Geometry: final body of the model. Coordinates: model frame, mm. Face numbers are marked on the shaded views. A direction names the side the tool comes from. Coordinates: 2 decimals unless noted, no trailing zeros. Order: outer loops, then holes, each group sorted by start corner. A loop starts at its lowest first (then second) coordinate and runs counter-clockwise, first axis right, second up. Notation, with made-up numbers: M 19,29 L 51,29 A14 ccw 51,52 Z; hole C 84,30.5 d10. An arc over 180 degrees is marked long. Use CSV: the item, a comma, the result in double quotes. Start each with the question number.
Q1. Section query C-C, the plane y = 33.5. Output: boundary loops of the cut face in (x, z).
Q2. Mould query, pull axis X, two halves, no side actions, for the marked faces 1, 2 and 3. Classes: +X half, -X half, draft (parallel to the pull), parting line (faces both ways), or undercut.
Q3. Access query for the marked faces 4 and 5. Directions: +Z, -Z, +X, -X, +Y, -Y. A direction counts if a zero-diameter tool reaches every point of the face in a straight line with its end or side. Return the directions, or none.
Q4. First-contact query: P1, Ø2.5, axis at x = 0, z = 0, coming from the +Y side; P2, Ø5, axis at x = 5.5, y = 20, coming from the +Z side; P3, Ø1, axis at y = 35, z = 2.5, coming from the +X side. Flat tips, straight axial feed; report the tip coordinate or a pass-through.
Q5. Section query D-D, the plane y = 14. Output: boundary loops of the cut face in (x, z), and give its area (3 significant figures).
Q6. Ray query, probe 1 along X at (y, z) = (34.25, 0); probe 2 along Y at (x, z) = (-7.75, 0.5); probe 3 along X at (y, z) = (2, 8). Return the intervals inside material, ascending.
Q7. Section query B-B, the plane x = 0. Output: boundary loops of the cut face in (y, z).
Q8. Section query A-A, the plane z = 0. Output: boundary loops of the cut face in (x, y), and give its area (3 significant figures).
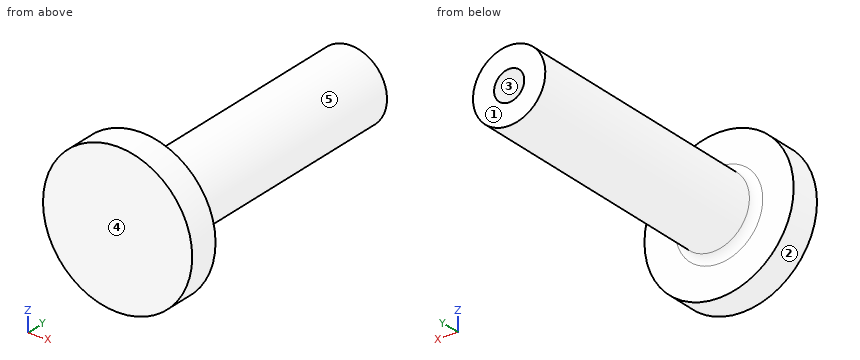
from build123d import *

# Parameters (mm, degrees)
SKETCH1_R           = 9.9
SKETCH1_R_2         = 4.8
SKETCH1_R_3         = 2
BOSS_EXTRUDE1_DEPTH = 4
BOSS_EXTRUDE2_START = 4
SKETCH1_3_R         = 4.8
SKETCH1_3_R_2       = 2
BOSS_EXTRUDE2_DEPTH = 36
CUT_EXTRUDE1_START  = 40
SKETCH1_4_R         = 2
CUT_EXTRUDE1_DEPTH  = 8
FILLET1_R           = 1


with BuildPart() as part:
    # Sketch1 → Boss-Extrude1 (new body)
    with BuildSketch(Plane(origin=(0, 0, 0), x_dir=(1, 0, 0), z_dir=(0, 1, 0))):
        with Locations(Location((0, 0, 0), (0, 0, 270))):
            Circle(SKETCH1_R)
        Circle(SKETCH1_R_2, mode=Mode.SUBTRACT)
        Circle(SKETCH1_R_2)
        Circle(SKETCH1_R_3, mode=Mode.SUBTRACT)
        Circle(SKETCH1_R_3)
    extrude(amount=BOSS_EXTRUDE1_DEPTH)

    # Sketch1<3> → Boss-Extrude2 (add)
    with BuildSketch(Plane(origin=(0, 0, 0), x_dir=(1, 0, 0), z_dir=(0, 1, 0)).offset(BOSS_EXTRUDE2_START)):
        with Locations(Location((0, 0, 0), (0, 0, 270))):
            Circle(SKETCH1_3_R)
        Circle(SKETCH1_3_R_2, mode=Mode.SUBTRACT)
        Circle(SKETCH1_3_R_2)
    extrude(amount=BOSS_EXTRUDE2_DEPTH)

    # Sketch1<4> → Cut-Extrude1 (cut)
    with BuildSketch(Plane(origin=(0, 0, 0), x_dir=(1, 0, 0), z_dir=(0, 1, 0)).offset(CUT_EXTRUDE1_START)):
        with Locations(Location((0, 0, 0), (0, 0, 270))):
            Circle(SKETCH1_4_R)
    extrude(amount=-CUT_EXTRUDE1_DEPTH, mode=Mode.SUBTRACT)

    # Fillet1
    fillet1_edges = [part.edges().sort_by_distance(p)[0] for p in [
        (0, 4, -4.8),
    ]]
    fillet(fillet1_edges, radius=FILLET1_R)


solid = part.part
Responses:
1,outline,"C 0,0 d9.6; hole C 0,0 d4"
2,face 1,"draft"
2,face 2,"parting line"
2,face 3,"undercut"
3,face 4,"+Z, -Z, +X, -X, -Y"
3,face 5,"+Y"
4,P1,"stops at y = 32"
4,P2,"stops at z = 3.75"
4,P3,"stops at x = 4.36"
5,outline,"C 0,0 d9.6"
5,area,"72.4 mm²"
6,probe 1,"x = -4.8 to -2, 2 to 4.8"
6,probe 2,"y = 0 to 4"
6,probe 3,"x = -5.83 to 5.83"
7,outline,"M 0,-9.9 L 4,-9.9 L 4,-5.8 A1 cw 5,-4.8 L 40,-4.8 L 40,-2 L 32,-2 L 32,2 L 40,2 L 40,4.8 L 5,4.8 A1 cw 4,5.8 L 4,9.9 L 0,9.9 Z"
8,outline,"M -9.9,0 L 9.9,0 L 9.9,4 L 5.8,4 A1 cw 4.8,5 L 4.8,40 L 2,40 L 2,32 L -2,32 L -2,40 L -4.8,40 L -4.8,5 A1 cw -5.8,4 L -9.9,4 Z"
8,area,"393 mm²"
